Work out the finished part from the listing and answer in its coordinate system (mm). Face numbers are marked on the shaded views. A direction names the side the tool comes from. Round coordinates to 2 decimals unless told otherwise and drop trailing zeros. Order: outer loops, then holes, each group sorted by start corner. A loop starts at its lowest first (then second) coordinate and runs counter-clockwise, first axis right, second up. Notation, with made-up numbers: M -16.75,-11 L 40.25,-11 A11 cw 40.25,3 Z; hole C 45,27 d10. An arc over 180 degrees is marked long. Return JSON: item names as keys, results as strings.
from build123d import *

# Parameters (mm, degrees)
CROQUIS1_W                 = 70
CROQUIS1_H                 = 62
SALIENTE_EXTRUIR1_DEPTH    = 3
CORTAR_EXTRUIR1_DEPTH      = 47.8508271
CORTAR_EXTRUIR2_DEPTH      = 47.8508271
CROQUIS4_W                 = 46
CROQUIS4_H                 = 10
CORTAR_EXTRUIR3_DEPTH      = 47.8508271
CROQUIS5_W                 = 46
CROQUIS5_H                 = 2
CORTAR_EXTRUIR4_DEPTH      = 47.8508271
CORTAR_EXTRUIR5_DEPTH      = 47.8508271
CORTAR_EXTRUIR5_DEPTH_BACK = 47.8508271
CROQUIS6_R                 = 1.625
CHAFL_N1_START             = -4
CHAFL_N1_OUTLINE_W         = 7.071067812
CHAFL_N1_OUTLINE_H         = 3
CHAFL_N1_DEPTH             = 4.707106781
CHAFL_N2_START             = -0.707106781
CHAFL_N2_OUTLINE_W         = 7.071067812
CHAFL_N2_OUTLINE_H         = 3
CHAFL_N2_DEPTH             = 4.707106781
CORTAR_EXTRUIR6_DEPTH      = 47.8508271
CORTAR_EXTRUIR6_DEPTH_BACK = 47.8508271
CROQUIS7_R                 = 8.25
SALIENTE_EXTRUIR2_DEPTH    = 3
CORTAR_EXTRUIR7_DEPTH      = 69.23672032
CORTAR_EXTRUIR7_DEPTH_BACK = 69.23672032
CORTAR_EXTRUIR8_DEPTH      = 47.8508271
CHAFL_N3_DEPTH             = 3
CHAFL_N5_DEPTH             = 3
CROQUIS13_W                = 50
CROQUIS13_H                = 30
SALIENTE_EXTRUIR3_DEPTH    = 3
CROQUIS14_W                = 50
CROQUIS14_H                = 30
SALIENTE_EXTRUIR4_DEPTH    = 3
REDONDEO1_R                = 5
CORTAR_EXTRUIR9_DEPTH      = 84.366660003
CORTAR_EXTRUIR9_DEPTH_BACK = 84.366660003
CROQUIS16_R                = 8.25
CROQUIS17_W                = 10.440463992
CROQUIS17_H                = 4.63729848
CORTAR_EXTRUIR10_DEPTH     = 5
CROQUIS18_W                = 0.779768004
CROQUIS18_H                = 2.68135076
SALIENTE_EXTRUIR5_DEPTH    = 3
CROQUIS19_W                = 0.779768004
CROQUIS19_H                = 2.68135076
SALIENTE_EXTRUIR6_DEPTH    = 3
REDONDEO6_R                = 3.5
REDONDEO7_R                = 3.5


with BuildPart() as part:
    # Croquis1 → Saliente-Extruir1 (new body)
    with BuildSketch(Plane(origin=(0, 0, 0), x_dir=(1, 0, 0), z_dir=(0, 1, 0))):
        Rectangle(CROQUIS1_W, CROQUIS1_H)
    extrude(amount=SALIENTE_EXTRUIR1_DEPTH)

    # Croquis2 → Cortar-Extruir1 (cut, through all)
    with BuildSketch(Plane(origin=(0, 3, 0), x_dir=(1, 0, 0), z_dir=(0, 1, 0))):
        Polygon((31.754264805, 31), (15.877132403, 58.5), (-15.877132403, 58.5), (-31.754264805, 31), (-15.877132403, 3.5), (15.877132403, 3.5), align=None)
    extrude(amount=-CORTAR_EXTRUIR1_DEPTH, mode=Mode.SUBTRACT)

    # Croquis3 → Cortar-Extruir2 (cut, through all)
    with BuildSketch(Plane(origin=(0, 3, 0), x_dir=(1, 0, 0), z_dir=(0, 1, 0))):
        with BuildLine():
            Line((-13, -21), (13, -21))
            ThreePointArc((13, -21), (23, -31), (13, -41))
            Line((13, -41), (-13, -41))
            ThreePointArc((-13, -41), (-23, -31), (-13, -21))
        make_face()
    extrude(amount=-CORTAR_EXTRUIR2_DEPTH, mode=Mode.SUBTRACT)

    # Croquis4 → Cortar-Extruir3 (cut, through all)
    with BuildSketch(Plane(origin=(0, 3, 0), x_dir=(1, 0, 0), z_dir=(0, 1, 0))):
        with Locations((0, -26)):
            Rectangle(CROQUIS4_W, CROQUIS4_H)
    extrude(amount=-CORTAR_EXTRUIR3_DEPTH, mode=Mode.SUBTRACT)

    # Croquis5 → Cortar-Extruir4 (cut, through all)
    with BuildSketch(Plane(origin=(0, 3, 0), x_dir=(1, 0, 0), z_dir=(0, 1, 0))):
        with Locations((0, -20)):
            Rectangle(CROQUIS5_W, CROQUIS5_H)
    extrude(amount=-CORTAR_EXTRUIR4_DEPTH, mode=Mode.SUBTRACT)

    # Croquis6 → Cortar-Extruir5 (cut, two sides: drawn at the far end of the back side and taken through both)
    with BuildSketch(Plane(origin=(0, 3, 0), x_dir=(1, 0, 0), z_dir=(0, 1, 0)).offset(-CORTAR_EXTRUIR5_DEPTH_BACK)):
        with Locations(Location((-29, -25.25, 0), (0, 0, 270))):
            Circle(CROQUIS6_R)
        with Locations(Location((29, -25.25, 0), (0, 0, 270))):
            Circle(CROQUIS6_R)
    extrude(amount=CORTAR_EXTRUIR5_DEPTH + CORTAR_EXTRUIR5_DEPTH_BACK, mode=Mode.SUBTRACT)

    # Chaflán1: read off the stored shape, not the designer's step
    # Chaflán1 outline → Chaflán1 (add)
    with BuildSketch(Plane(origin=(0, 0, 0), x_dir=(0.7071067811865471, 0, -0.707106781186548), z_dir=(0.707106781186548, 0, 0.707106781186547)).offset(CHAFL_N1_START)):
        with Locations((-29.69848481, 1.5)):
            Rectangle(CHAFL_N1_OUTLINE_W, CHAFL_N1_OUTLINE_H)
    extrude(amount=CHAFL_N1_DEPTH)

    # Chaflán2: read off the stored shape, not the designer's step
    # Chaflán2 outline → Chaflán2 (add)
    with BuildSketch(Plane(origin=(0, 0, 0), x_dir=(0.707106781186548, 0, 0.707106781186547), z_dir=(0.707106781186547, 0, -0.707106781186548)).offset(CHAFL_N2_START)):
        with Locations((29.69848481, -1.5)):
            Rectangle(CHAFL_N2_OUTLINE_W, CHAFL_N2_OUTLINE_H)
    extrude(amount=CHAFL_N2_DEPTH)

    # Croquis7 → Cortar-Extruir6 (cut, two sides: drawn at the far end of the back side and taken through both)
    with BuildSketch(Plane(origin=(0, 3, 0), x_dir=(1, 0, 0), z_dir=(0, 1, 0)).offset(-CORTAR_EXTRUIR6_DEPTH_BACK)):
        with Locations(Location((-12.93, -6.5, 0), (0, 0, 270))):
            Circle(CROQUIS7_R)
        with Locations(Location((12.93, -6.5, 0), (0, 0, 270))):
            Circle(CROQUIS7_R)
    extrude(amount=CORTAR_EXTRUIR6_DEPTH + CORTAR_EXTRUIR6_DEPTH_BACK, mode=Mode.SUBTRACT)

    # Croquis8 → Saliente-Extruir2 (add)
    with BuildSketch(Plane(origin=(0, 3, 0), x_dir=(1, 0, 0), z_dir=(0, 1, 0))):
        Polygon((15.877132403, 3.5), (31.754264805, 31), (15.877132403, 58.5), (-15.877132403, 58.5), (-31.754264805, 31), (-15.877132403, 3.5), (0, 3.5), align=None)
    extrude(amount=-SALIENTE_EXTRUIR2_DEPTH)

    # Croquis9 → Cortar-Extruir7 (cut, two sides: drawn at the far end of the back side and taken through both)
    with BuildSketch(Plane(origin=(0, 3, 0), x_dir=(1, 0, 0), z_dir=(0, 1, 0)).offset(-CORTAR_EXTRUIR7_DEPTH_BACK)):
        Polygon((-232.018715641, 31), (-35, 31), (35, 31), (232.018715641, 31), (232.018715641, 425.037431282), (-232.018715641, 425.037431282), align=None)
    extrude(amount=CORTAR_EXTRUIR7_DEPTH + CORTAR_EXTRUIR7_DEPTH_BACK, mode=Mode.SUBTRACT)

    # Croquis10 → Cortar-Extruir8 (cut, through all)
    with BuildSketch(Plane(origin=(0, 3, 0), x_dir=(1, 0, 0), z_dir=(0, 1, 0))):
        Polygon((0, 6), (-32, 6), (-32, 31), (32, 31), (32, 6), align=None)
    extrude(amount=-CORTAR_EXTRUIR8_DEPTH, mode=Mode.SUBTRACT)

    # Chaflán3: read off the stored shape, not the designer's step
    # Chaflán3 outline → Chaflán3 (add)
    with BuildSketch(Plane(origin=(0, 0, 0), x_dir=(1, 0, 0), z_dir=(0, 1, 0))):
        Polygon((-32, 6), (-17, 6), (-32, 31), align=None)
    extrude(amount=CHAFL_N3_DEPTH)

    # Chaflán5: read off the stored shape, not the designer's step
    # Chaflán5 outline → Chaflán5 (add)
    with BuildSketch(Plane(origin=(0, 0, 0), x_dir=(1, 0, 0), z_dir=(0, 1, 0))):
        Polygon((32, 6), (32, 31), (17, 6), align=None)
    extrude(amount=CHAFL_N5_DEPTH)

    # Croquis13 → Saliente-Extruir3 (add)
    with BuildSketch(Plane.ZY.offset(35)):
        with Locations((-6, 18)):
            Rectangle(CROQUIS13_W, CROQUIS13_H)
    extrude(amount=-SALIENTE_EXTRUIR3_DEPTH)

    # Croquis14 → Saliente-Extruir4 (add)
    with BuildSketch(Plane(origin=(35, 0, 0), x_dir=(0, 0, -1), z_dir=(1, 0, 0))):
        with Locations((6, 18)):
            Rectangle(CROQUIS14_W, CROQUIS14_H)
    extrude(amount=-SALIENTE_EXTRUIR4_DEPTH)

    # Redondeo1
    redondeo1_edges = [part.edges().sort_by_distance(p)[0] for p in [
        (-23, 1.5, 31),
        (23, 1.5, 31),
        (35, 1.5, 31),
        (-35, 1.5, 31),
    ]]
    fillet(redondeo1_edges, radius=REDONDEO1_R)

    # Croquis16 → Cortar-Extruir9 (cut, two sides: drawn at the far end of the back side and taken through both)
    with BuildSketch(Plane.ZY.offset(35).offset(-CORTAR_EXTRUIR9_DEPTH_BACK)):
        with Locations((-18.93, 20.5)):
            Circle(CROQUIS16_R)
        with Locations((6.92, 20.5)):
            Circle(CROQUIS16_R)
    extrude(amount=CORTAR_EXTRUIR9_DEPTH + CORTAR_EXTRUIR9_DEPTH_BACK, mode=Mode.SUBTRACT)

    # Croquis17 → Cortar-Extruir10 (cut)
    with BuildSketch(Plane(origin=(0, 3, 0), x_dir=(1, 0, 0), z_dir=(0, 1, 0))):
        with Locations((-29, -31)):
            Rectangle(CROQUIS17_W, CROQUIS17_H)
        with Locations((29, -31)):
            Rectangle(CROQUIS17_W, CROQUIS17_H)
    extrude(amount=-CORTAR_EXTRUIR10_DEPTH, mode=Mode.SUBTRACT)

    # Croquis18 → Saliente-Extruir5 (add)
    with BuildSketch(Plane(origin=(0, 3, 0), x_dir=(1, 0, 0), z_dir=(0, 1, 0))):
        with Locations((-34.610115998, -27.34067538)):
            Rectangle(CROQUIS18_W, CROQUIS18_H)
        with Locations((-23.389884002, -27.34067538)):
            Rectangle(CROQUIS18_W, CROQUIS18_H)
    extrude(amount=-SALIENTE_EXTRUIR5_DEPTH)

    # Croquis19 → Saliente-Extruir6 (add)
    with BuildSketch(Plane(origin=(0, 3, 0), x_dir=(1, 0, 0), z_dir=(0, 1, 0))):
        with Locations((23.389884002, -27.34067538)):
            Rectangle(CROQUIS19_W, CROQUIS19_H)
        with Locations((34.610115998, -27.34067538)):
            Rectangle(CROQUIS19_W, CROQUIS19_H)
    extrude(amount=-SALIENTE_EXTRUIR6_DEPTH)

    # Redondeo6
    redondeo6_edges = [part.edges().sort_by_distance(p)[0] for p in [
        (-35, 1.5, 28.68135076),
    ]]
    fillet(redondeo6_edges, radius=REDONDEO6_R)

    # Redondeo7
    redondeo7_edges = [part.edges().sort_by_distance(p)[0] for p in [
        (-23, 1.5, 28.68135076),
        (23, 1.5, 28.68135076),
        (35, 1.5, 28.68135076),
    ]]
    fillet(redondeo7_edges, radius=REDONDEO7_R)


solid = part.part
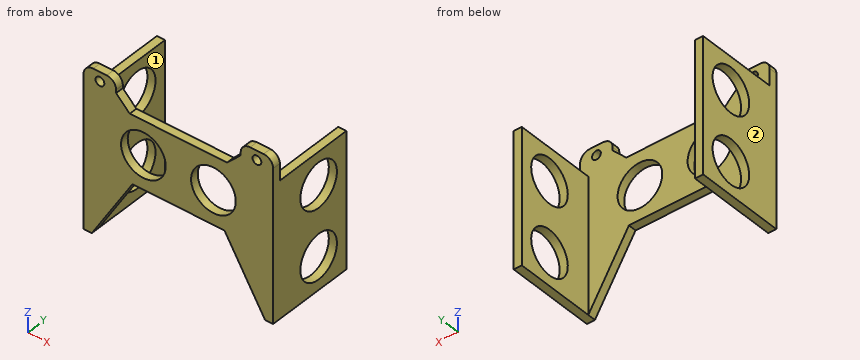
Item 1: Each of these flat-tipped pins is pushed along its axis until it touches: pin 1 (15 mm diameter, centred on y = 20.5, z = -18.93, fed in from +X); pin 2 (2.5 mm diameter, centred on x = 33.5, y = 19.5, fed in from +Z); pin 3 (1.5 mm diameter, centred on x = -2, y = 1, fed in from -Z); pin 4 (5 mm diameter, centred on x = 8, z = -1, fed in from +Y). Where does it stop, or does it pass through?
Output:
{"pin 1": "passes through", "pin 2": "stops at z = 19", "pin 3": "stops at z = -6", "pin 4": "stops at y = 3"}
Item 2: Find section A-A (x = 29). Determine the outline of the cut face in (y, z) (3 decimals).
Output:
{"outline": "M 0,-26 L 3,-26 L 3,23.625 L 0,23.625 Z; M 0,26.875 L 3,26.875 L 3,28.681 L 0,28.681 Z"}
Item 3: Which of the six approach directions +Z, -Z, +X, -X, +Y, -Y give full straight-line access (tool end or side, diameter ignored) to the marked faces 1 and 2?
Output:
{"face 1": "+Z, -Z, +Y", "face 2": "+Z, -Z, -X, +Y, -Y"}
Item 4: Find section D-D (z = -18.93). Determine the outline of the cut face in (x, y).
Output:
{"outline": "M -35,0 L -24.76,0 L -24.76,3 L -32,3 L -32,12.25 L -35,12.25 Z; M -35,28.75 L -32,28.75 L -32,33 L -35,33 Z; M 24.76,0 L 35,0 L 35,12.25 L 32,12.25 L 32,3 L 24.76,3 Z; M 32,28.75 L 35,28.75 L 35,33 L 32,33 Z"}
Item 5: Consider line 1 along X through (y, z) = (1.6, 25.25) (3 decimals); line 2 along X through (y, z) = (1.45, 6.5); line 3 along X through (y, z) = (5.5, 4). Determine where each line is inside the solid, lowest interval first. Write a range as [from, to].
Output:
{"line 1": "x = [-34.999, -30.625], [-27.375, -23.001], [23.001, 27.375], [30.625, 34.999]", "line 2": "x = [-35, -21.18], [-4.68, 4.68], [21.18, 35]", "line 3": "x = [-35, -32], [32, 35]"}
Item 6: Find section C-C (y = 20.5). Determine the outline of the cut face in (x, z), plus the area to 3 significant figures.
Output:
{"outline": "M -35,-31 L -32,-31 L -32,-27.18 L -35,-27.18 Z; M -35,-10.68 L -32,-10.68 L -32,-1.33 L -35,-1.33 Z; M -35,15.17 L -32,15.17 L -32,19 L -35,19 Z; M 32,-31 L 35,-31 L 35,-27.18 L 32,-27.18 Z; M 32,-10.68 L 35,-10.68 L 35,-1.33 L 32,-1.33 Z; M 32,15.17 L 35,15.17 L 35,19 L 32,19 Z", "area": "102 mm^2"}
Item 7: Find section B-B (y = 31). Determine the outline of the cut face in (x, z), plus the area to 3 significant figures.
Output:
{"outline": "M -35,-31 L -32,-31 L -32,19 L -35,19 Z; M 32,-31 L 35,-31 L 35,19 L 32,19 Z", "area": "300 mm^2"}
